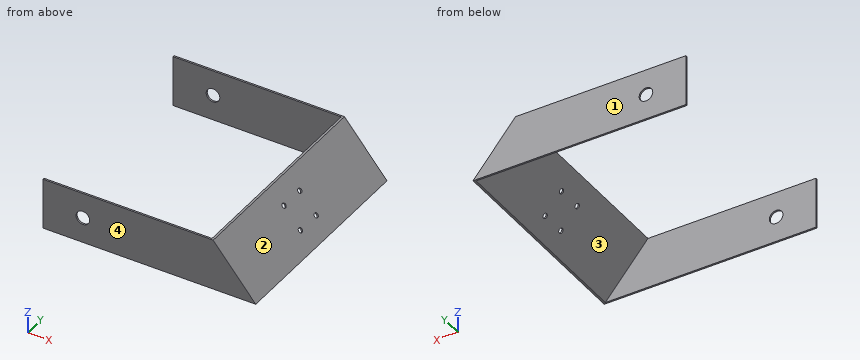
from build123d import *

# Parameters (mm, degrees)
SKETCH1_W           = 125
SKETCH1_H           = 125
BOSS_EXTRUDE1_DEPTH = 30
CUT_EXTRUDE1_DEPTH  = 125
SHELL1_T            = -1
SKETCH3_R           = 4
CUT_EXTRUDE2_DEPTH  = 125
CUT_EXTRUDE3_DEPTH  = 125


with BuildPart() as part:
    # Sketch1 → Boss-Extrude1 (new body)
    with BuildSketch(Plane.XY):
        with Locations((62.5, 62.5)):
            Rectangle(SKETCH1_W, SKETCH1_H)
    extrude(amount=BOSS_EXTRUDE1_DEPTH)

    # Sketch2 → Cut-Extrude1 (cut)
    with BuildSketch(Plane(origin=(0, 125, 0), x_dir=(1, 0, 0), z_dir=(0, 1, 0))):
        Polygon((125, 0), (100, -30), (125, -30), align=None)
    extrude(amount=-CUT_EXTRUDE1_DEPTH, mode=Mode.SUBTRACT)

    # Shell1
    shell1_openings = [part.faces().sort_by_distance(p)[0] for p in [
        (50, 62.5, 30),
        (62.5, 62.5, 0),
        (0, 62.5, 15),
    ]]
    offset(amount=SHELL1_T, openings=shell1_openings, kind=Kind.INTERSECTION)

    # Sketch3 → Cut-Extrude2 (cut)
    with BuildSketch(Plane(origin=(0, 0, 0), x_dir=(-1, 0, 0), z_dir=(0, -1, 0))):
        with Locations(Location((-23.380174368, -15, 0), (0, 0, 90))):
            Circle(SKETCH3_R)
    extrude(amount=-CUT_EXTRUDE2_DEPTH, mode=Mode.SUBTRACT)

    # Sketch4 → Cut-Extrude3 (cut)
    with BuildSketch(Plane(origin=(73.770491803, 0, 61.475409836), x_dir=(0.6401843996644799, 0, -0.7682212795973759), z_dir=(0.768221279597376, 0, 0.6401843996644799))):
        with BuildLine():
            Line((52.997425768, 68.55), (52.997425768, 70))
            Line((52.997425768, 70), (54.447425768, 70))
            ThreePointArc((54.447425768, 70), (51.972120936, 71.025304833), (52.997425768, 68.55))
        make_face()
        with BuildLine():
            Line((54.447425768, 70), (52.997425768, 70))
            Line((52.997425768, 70), (52.997425768, 68.55))
            ThreePointArc((52.997425768, 68.55), (54.022730601, 68.974695167), (54.447425768, 70))
        make_face()
        with BuildLine():
            ThreePointArc((69.447425768, 70), (67.997425768, 71.45), (66.547425768, 70))
            Line((66.547425768, 70), (67.997425768, 70))
            Line((67.997425768, 70), (67.997425768, 68.55))
            ThreePointArc((67.997425768, 68.55), (69.022730601, 68.974695167), (69.447425768, 70))
        make_face()
        with BuildLine():
            Line((67.997425768, 70), (66.547425768, 70))
            ThreePointArc((66.547425768, 70), (66.972120936, 68.974695167), (67.997425768, 68.55))
            Line((67.997425768, 68.55), (67.997425768, 70))
        make_face()
        with BuildLine():
            ThreePointArc((54.447425768, 55), (54.022730601, 56.025304833), (52.997425768, 56.45))
            Line((52.997425768, 56.45), (52.997425768, 55))
            Line((52.997425768, 55), (54.447425768, 55))
        make_face()
        with BuildLine():
            Line((52.997425768, 55), (52.997425768, 56.45))
            ThreePointArc((52.997425768, 56.45), (51.972120936, 53.974695167), (54.447425768, 55))
            Line((54.447425768, 55), (52.997425768, 55))
        make_face()
        with BuildLine():
            ThreePointArc((69.447425768, 55), (69.022730601, 56.025304833), (67.997425768, 56.45))
            Line((67.997425768, 56.45), (67.997425768, 55))
            Line((67.997425768, 55), (66.547425768, 55))
            ThreePointArc((66.547425768, 55), (67.997425768, 53.55), (69.447425768, 55))
        make_face()
        with BuildLine():
            Line((67.997425768, 55), (67.997425768, 56.45))
            ThreePointArc((67.997425768, 56.45), (66.972120936, 56.025304833), (66.547425768, 55))
            Line((66.547425768, 55), (67.997425768, 55))
        make_face()
    extrude(amount=-CUT_EXTRUDE3_DEPTH, mode=Mode.SUBTRACT)


solid = part.part
Verification items for the finished model (mm, model axes). Face numbers are marked on the shaded views. Coordinates: 2 decimals unless noted, no trailing zeros. Write each loop counter-clockwise with the first axis right and the second up, starting at its lowest first coordinate (ties: lowest second). Pieces come first, ordered by that corner, then holes. Notation, with made-up numbers: M 4.5,32 L 45.5,32 A32 ccw 45.5,68 Z; hole C -3,61.5 d11. An arc over 180 degrees is marked long. One line per question, with ' | ' between items.
1) Sectioned sample at C-C on y = 103. Record the cut outline in (x, z).
Solutions:
outline: M 98.7,30 L 123.7,0 L 125,0 L 100,30 Z
2) Sectioned sample at A-A on x = 66.5. Record the cut outline in (y, z).
Solutions:
outline: M 0,0 L 1,0 L 1,30 L 0,30 Z; M 124,0 L 125,0 L 125,30 L 124,30 Z
3) Material ranges on L1, parallel to Y at x = 52, z = 11.5; L2, parallel to X at y = 0.55, z = 15; L3, parallel to X at y = 11, z = 14.5, recorded low to high.
Solutions:
L1: 0 to 1, 124 to 125 | L2: 0 to 19.38, 27.38 to 112.5 | L3: 111.61 to 112.92
4) Release check for a two-part mould opening along Y. For the marked faces 1, 2, 3 and 4 record: +Y half, -Y half, draft (parallel to the pull), parting line (faces both ways), or undercut.
Solutions:
face 1: +Y half | face 2: draft | face 3: undercut | face 4: -Y half
5) Sectioned sample at B-B on z = 15. Record the cut outline in (x, y).
Solutions:
outline: M 0,0 L 19.38,0 L 19.38,1 L 0,1 Z; M 0,124 L 19.38,124 L 19.38,125 L 0,125 Z; M 27.38,0 L 112.5,0 L 112.5,125 L 27.38,125 L 27.38,124 L 111.2,124 L 111.2,1 L 27.38,1 Z
6) Sectioned sample at D-D on x = 102.5. Record the cut outline in (y, z).
Solutions:
outline: M 0,0 L 1,0 L 1,25.44 L 124,25.44 L 124,0 L 125,0 L 125,27 L 0,27 Z
7) Depth check by flat-ended pin: pin 1 Ø3 at (y, z) = (63.5, 9) entering from -X; pin 2 Ø1.5 at (x, z) = (30.5, 24.5) entering from -Y; pin 3 Ø7 at (x, z) = (23.38, 15) entering from -Y. Enter the tip coordinate at first touch or a pass-through.
Solutions:
pin 1: x = 114.95 | pin 2: y = 0 | pin 3: through
